```python
from build123d import *

# Parameters (mm, degrees)
SKETCH1_W           = 21
SKETCH1_H           = 21
BOSS_EXTRUDE1_DEPTH = 8
FILLET1_R           = 5
CUT_EXTRUDE2_DEPTH  = 6.5
SKETCH11_R          = 2.65
BOSS_EXTRUDE4_DEPTH = 3
SKETCH2_R           = 5


with BuildPart() as part:
    # Sketch1 → Boss-Extrude1 (new body)
    with BuildSketch(Plane(origin=(0, 0, 0), x_dir=(1, 0, 0), z_dir=(0, 1, 0))):
        with Locations((10.5, -10.5)):
            Rectangle(SKETCH1_W, SKETCH1_H)
    extrude(amount=BOSS_EXTRUDE1_DEPTH)

    # Fillet1
    fillet1_edges = [part.edges().sort_by_distance(p)[0] for p in [
        (0, 4, 0),
        (21, 4, 0),
        (21, 4, 21),
        (0, 4, 21),
    ]]
    fillet(fillet1_edges, radius=FILLET1_R)

    # Sketch10 → Cut-Extrude2 (cut)
    with BuildSketch(Plane.XZ):
        with BuildLine():
            Line((5, 1.5), (16, 1.5))
            ThreePointArc((16, 1.5), (18.474873734, 2.525126266), (19.5, 5))
            Line((19.5, 5), (19.5, 16))
            ThreePointArc((19.5, 16), (18.474873734, 18.474873734), (16, 19.5))
            Line((16, 19.5), (5, 19.5))
            ThreePointArc((5, 19.5), (2.525126266, 18.474873734), (1.5, 16))
            Line((1.5, 16), (1.5, 5))
            ThreePointArc((1.5, 5), (2.525126266, 2.525126266), (5, 1.5))
        make_face()
    extrude(amount=-CUT_EXTRUDE2_DEPTH, mode=Mode.SUBTRACT)

    # Sketch11 → Boss-Extrude4 (add)
    with BuildSketch(Plane.XZ.offset(-6.5)):
        with Locations(Location((10.5, 10.5, 0), (0, 0, 90))):
            Circle(SKETCH11_R)
    extrude(amount=BOSS_EXTRUDE4_DEPTH)

    # Sketch3 → Loft2 section 0
    with BuildSketch(Plane(origin=(0, 8, 0), x_dir=(1, 0, 0), z_dir=(0, 1, 0))):
        with BuildLine():
            Line((16, 0), (5, 0))
            ThreePointArc((5, 0), (1.464466094, -1.464466094), (0, -5))
            Line((0, -5), (0, -16))
            ThreePointArc((0, -16), (1.464466094, -19.535533906), (5, -21))
            Line((5, -21), (16, -21))
            ThreePointArc((16, -21), (19.535533906, -19.535533906), (21, -16))
            Line((21, -16), (21, -5))
            ThreePointArc((21, -5), (19.535533906, -1.464466094), (16, 0))
        make_face()
    # Sketch2 → Loft2 section 1
    with BuildSketch(Plane(origin=(0, 9.5, 0), x_dir=(1, 0, 0), z_dir=(0, 1, 0))):
        with Locations((10.5, -10.5)):
            Circle(SKETCH2_R)
    loft()


solid = part.part
```
Source: CAD feature listing. Evaluate the final solid. Frame: model axes, mm. A direction names the side the tool comes from. Give positions to 0.01 mm unless a question says otherwise; leave off trailing zeros. Loops run counter-clockwise (first coordinate to the right, second up) from the corner with the lowest first, then second, coordinate; pieces in that order, holes last. Notation, with made-up numbers: (-12, 22) -> (11, 22) arc R17 cw to (11, 51) -> close; hole circle Ø1 at (-38, -28). An arc over 180 degrees is marked (long way). Use a Markdown table: item, result. Add a question column.
(1) Pull-direction query (X, two-part tool) for faces 3 (the face through (1, 4, 2)), 4 (the face through (11, 3, 19.5)), 5 (the face through (10, 4, 21)); classes: +X half, -X half, draft (parallel to the pull), parting line (faces both ways), or undercut.
(2) Section query B-B (y = 1.5). Output: boundary loops of the cut face in (x, z).
(3) Access query for faces 1 (the face through (13.09, 5.02, 9.93)), 2 (the face through (19, 4, 20)). Directions: +Z, -Z, +X, -X, +Y, -Y. A direction counts if a zero-diameter tool reaches every point of the face in a straight line with its end or side. Return the directions, or none.
(4) Section query A-A (y = 4.5). Output: boundary loops of the cut face in (x, z), then the cut area to 3 significant figures.
(5) Ray query, line 1 (Z direction, x = 11.25, y = 3.75); line 2 (X direction, y = 2.5, z = 13.25); line 3 (X direction, y = 5.5, z = 12.25). Return the intervals inside material, ascending.
(6) First-contact query: pin 1 Ø6 at (x, z) = (17.5, 10) entering from -Y; pin 2 Ø1.5 at (x, z) = (2.5, 9.5) entering from -Y; pin 3 Ø1.6 at (x, z) = (10, 11.5) entering from -Y. Flat tips, straight axial feed; report the tip coordinate or a pass-through.
Checked values:
| question | item | result |
|---|---|---|
| 1 | face 3 | -X half |
| 1 | face 4 | undercut |
| 1 | face 5 | draft |
| 2 | outline | (0, 5) arc R5 ccw to (5, 0) -> (16, 0) arc R5 ccw to (21, 5) -> (21, 16) arc R5 ccw to (16, 21) -> (5, 21) arc R5 ccw to (0, 16) -> close; hole (1.5, 5) arc R3.5 ccw to (5, 1.5) -> (16, 1.5) arc R3.5 ccw to (19.5, 5) -> (19.5, 16) arc R3.5 ccw to (16, 19.5) -> (5, 19.5) arc R3.5 ccw to (1.5, 16) -> close |
| 3 | face 1 | -Y |
| 3 | face 2 | +Z, +X, +Y, -Y |
| 4 | outline | (0, 5) arc R5 ccw to (5, 0) -> (16, 0) arc R5 ccw to (21, 5) -> (21, 16) arc R5 ccw to (16, 21) -> (5, 21) arc R5 ccw to (0, 16) -> close; circle Ø5.3 at (10.5, 10.5); hole (1.5, 5) arc R3.5 ccw to (5, 1.5) -> (16, 1.5) arc R3.5 ccw to (19.5, 5) -> (19.5, 16) arc R3.5 ccw to (16, 19.5) -> (5, 19.5) arc R3.5 ccw to (1.5, 16) -> close |
| 4 | area | 128 mm^2 |
| 5 | line 1 | 0 to 1.5, 7.96 to 13.04, 19.5 to 21 |
| 5 | line 2 | 0 to 1.5, 19.5 to 21 |
| 5 | line 3 | 0 to 1.5, 8.51 to 12.49, 19.5 to 21 |
| 6 | pin 1 | y = 0 |
| 6 | pin 2 | y = 6.5 |
| 6 | pin 3 | y = 3.5 |
